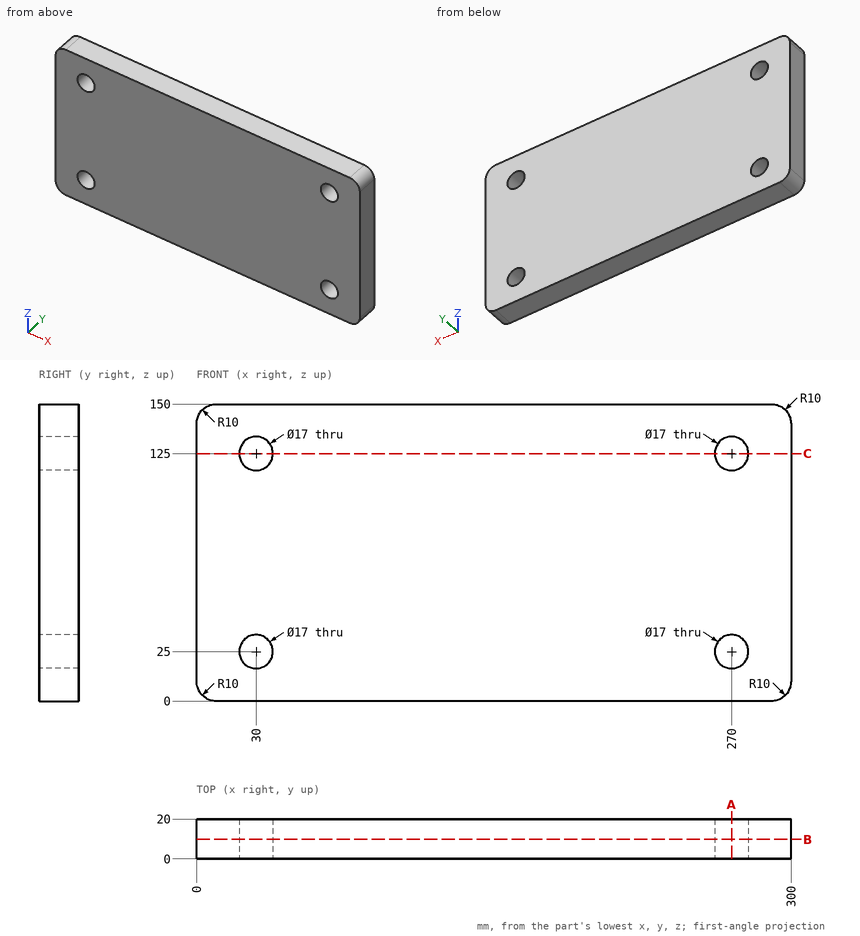
Here's the drawing with two shaded views (mm, measured from the low corner). I have some questions. Coordinates: 2 decimals unless noted, no trailing zeros. Loops run counter-clockwise (first coordinate to the right, second up) from the corner with the lowest first, then second, coordinate; pieces in that order, holes last. Notation, with made-up numbers: M -21,45 L 13,45 A12 ccw 13,58 Z; hole C 51,57.25 d1. An arc over 180 degrees is marked long. Put each result on its own line as item: value. Start each with the question number.
(1) Will this pin go through, and if not, where does the flat tip stop? pin 1 Ø10 at (x, z) = (270, 125) entering from +Y.
(2) Imagine slicing it at C-C on z = 125. List the corners of the cut face in (x, y) for me, and give its area (3 significant figures).
(3) Imagine slicing it at B-B on y = 9.75. List the corners of the cut face in (x, z) for me.
(4) I need wall thicknesses on probe 1 along X at (y, z) = (10, 125); probe 2 along Z at (x, y) = (270, 11.75); probe 3 along Z at (x, y) = (274, 5.75). Which ranges of each line are inside material? Lowest first, please.
(5) Imagine slicing it at A-A on x = 270. List the corners of the cut face in (y, z) for me, and give its area (3 significant figures).
Worked answers:
1. pin 1: passes through
2. outline: M 0,0 L 21.5,0 L 21.5,20 L 0,20 Z; M 38.5,0 L 261.5,0 L 261.5,20 L 38.5,20 Z; M 278.5,0 L 300,0 L 300,20 L 278.5,20 Z
2. area: 5,320 mm2
3. outline: M 0,10 A10 ccw 10,0 L 290,0 A10 ccw 300,10 L 300,140 A10 ccw 290,150 L 10,150 A10 ccw 0,140 Z; hole C 30,25 d17; hole C 30,125 d17; hole C 270,25 d17; hole C 270,125 d17
4. probe 1: x = 0 to 21.5, 38.5 to 261.5, 278.5 to 300
4. probe 2: z = 0 to 16.5, 33.5 to 116.5, 133.5 to 150
4. probe 3: z = 0 to 17.5, 32.5 to 117.5, 132.5 to 150
5. outline: M 0,0 L 20,0 L 20,16.5 L 0,16.5 Z; M 0,33.5 L 20,33.5 L 20,116.5 L 0,116.5 Z; M 0,133.5 L 20,133.5 L 20,150 L 0,150 Z
5. area: 2,320 mm2
